The listing builds one solid part. Answer for the finished solid, in the listing's coordinates (mm). A direction names the side the tool comes from. Coordinates: 2 decimals unless noted, no trailing zeros. Write each loop counter-clockwise with the first axis right and the second up, starting at its lowest first coordinate (ties: lowest second). Pieces come first, ordered by that corner, then holes.
from build123d import *

# Parameters (mm, degrees)
MODEL_R                 = 1.5
SALIENTE_EXTRUIR1_DEPTH = 3


with BuildPart() as part:
    # Model → Saliente-Extruir1 (new body)
    with BuildSketch(Plane.XY):
        with BuildLine():
            Line((174.227054575, 213.178720063), (174.227054575, 204.178720063))
            ThreePointArc((174.227054575, 204.178720063), (174.569596678, 202.456644617), (175.545074059, 200.996739548))
            Line((175.545074059, 200.996739548), (184.545074059, 191.996739548))
            ThreePointArc((184.545074059, 191.996739548), (187.727054575, 190.678720063), (190.90903509, 191.996739548))
            Line((190.90903509, 191.996739548), (199.90903509, 200.996739548))
            ThreePointArc((199.90903509, 200.996739548), (200.884512471, 202.456644617), (201.227054575, 204.178720063))
            Line((201.227054575, 204.178720063), (201.227054575, 217.678720063))
            Line((201.227054575, 217.678720063), (174.227054575, 217.678720063))
            Line((174.227054575, 217.678720063), (174.227054575, 213.178720063))
        make_face()
        with Locations((187.727054575, 204.178720063)):
            Circle(MODEL_R, mode=Mode.SUBTRACT)
        with Locations((178.727054575, 204.178720063)):
            Circle(MODEL_R, mode=Mode.SUBTRACT)
        with Locations((187.727054575, 213.178720063)):
            Circle(MODEL_R, mode=Mode.SUBTRACT)
        with Locations((187.727054575, 195.178720063)):
            Circle(MODEL_R, mode=Mode.SUBTRACT)
        with Locations((196.727054575, 204.178720063)):
            Circle(MODEL_R, mode=Mode.SUBTRACT)
        with BuildLine():
            Line((193.477054575, 214.053720063), (193.477054575, 212.303720063))
            ThreePointArc((193.477054575, 212.303720063), (193.696724489, 211.773389977), (194.227054575, 211.553720063))
            Line((194.227054575, 211.553720063), (199.227054575, 211.553720063))
            ThreePointArc((199.227054575, 211.553720063), (199.757384661, 211.773389977), (199.977054575, 212.303720063))
            Line((199.977054575, 212.303720063), (199.977054575, 214.053720063))
            ThreePointArc((199.977054575, 214.053720063), (199.757384661, 214.584050149), (199.227054575, 214.803720063))
            Line((199.227054575, 214.803720063), (194.227054575, 214.803720063))
            ThreePointArc((194.227054575, 214.803720063), (193.696724489, 214.584050149), (193.477054575, 214.053720063))
        make_face(mode=Mode.SUBTRACT)
        with BuildLine():
            Line((175.477054575, 214.053720063), (175.477054575, 212.303720063))
            ThreePointArc((175.477054575, 212.303720063), (175.696724489, 211.773389977), (176.227054575, 211.553720063))
            Line((176.227054575, 211.553720063), (181.227054575, 211.553720063))
            ThreePointArc((181.227054575, 211.553720063), (181.757384661, 211.773389977), (181.977054575, 212.303720063))
            Line((181.977054575, 212.303720063), (181.977054575, 214.053720063))
            ThreePointArc((181.977054575, 214.053720063), (181.757384661, 214.584050149), (181.227054575, 214.803720063))
            Line((181.227054575, 214.803720063), (176.227054575, 214.803720063))
            ThreePointArc((176.227054575, 214.803720063), (175.696724489, 214.584050149), (175.477054575, 214.053720063))
        make_face(mode=Mode.SUBTRACT)
    extrude(amount=SALIENTE_EXTRUIR1_DEPTH)


solid = part.part
Q1. Find the intervals of material crossed by probe 1 along X at (y, z) = (213.5, 0.7); probe 2 along Y at (x, z) = (187.25, 2.7); probe 3 along Y at (x, z) = (195.75, 0.9), in increasing order.
Answers below:
probe 1: x = 174.23 to 175.48, 181.98 to 186.26, 189.19 to 193.48, 199.98 to 201.23
probe 2: y = 190.7 to 193.76, 196.6 to 202.76, 205.6 to 211.76, 214.6 to 217.68
probe 3: y = 196.84 to 203.04, 205.32 to 211.55, 214.8 to 217.68
Q2. Which of the six approach directions +Z, -Z, +X, -X, +Y, -Y give full straight-line access (tool end or side, diameter ignored) to faces 1 (the face through (181.977, 213, 1)), 2 (the face through (188, 207, 0))?
Answers below:
face 1: +Z, -Z
face 2: -Z, +X, -X, +Y, -Y
Q3. Given pin 1 (2 mm diameter, centred on x = 182.5, y = 194, fed in from +Z); pin 2 (1.5 mm diameter, centred on x = 195.5, z = 2, fed in from -Y); pin 3 (0.9 mm diameter, centred on x = 179.5, z = 1, fed in from -Y), each flat-ended and moving along its own axis, determine where each tip first touches the part or whether it passes through.
Answers below:
pin 1: stops at z = 3
pin 2: stops at y = 195.84
pin 3: stops at y = 196.59
Q4. The part is cut by section C-C, the plane x = 197. Write down the section's boundary in (y, z).
Answers below:
outline: (198.09, 0) - (202.7, 0) - (202.7, 3) - (198.09, 3) - close; (205.65, 0) - (211.55, 0) - (211.55, 3) - (205.65, 3) - close; (214.8, 0) - (217.68, 0) - (217.68, 3) - (214.8, 3) - close
Q5. The part is cut by section A-A, the plane y = 203.25. Write down the section's boundary in (x, z).
Answers below:
outline: (174.32, 0) - (177.55, 0) - (177.55, 3) - (174.32, 3) - close; (179.9, 0) - (186.55, 0) - (186.55, 3) - (179.9, 3) - close; (188.9, 0) - (195.55, 0) - (195.55, 3) - (188.9, 3) - close; (197.9, 0) - (201.13, 0) - (201.13, 3) - (197.9, 3) - close
Q6. Determine the mould class of faces 3 (the face through (180.158, 204.629, 1.479)), 4 (the face through (201.227, 211, 1)), 5 (the face through (188, 217.679, 1)) for opening direction X: released by +X, released by -X, zero draft, split by the parting line, or undercut.
Answers below:
face 3: undercut
face 4: released by +X
face 5: zero draft
Q7. The part is cut by section D-D, the plane y = 199.25. Write down the section's boundary in (x, z).
Answers below:
outline: (177.29, 0) - (198.16, 0) - (198.16, 3) - (177.29, 3) - close
Q8. The part is cut by section B-B, the plane z = 0.4. State how many separate pieces and enclosed holes the cut face has, then the cut area to 3 significant figures.
Answers below:
separate pieces: 1
enclosed holes: 7
area: 515 mm2
